```python
from build123d import *

# Parameters (mm, degrees)
SKETCH1_R           = 2.25
BOSS_EXTRUDE1_DEPTH = 3
BOSS_EXTRUDE2_DEPTH = 40
BOSS_EXTRUDE3_START = -2
BOSS_EXTRUDE3_DEPTH = 3
SKETCH6_R           = 1.5
CUT_EXTRUDE1_DEPTH  = 39
FILLET1_R           = 2


with BuildPart() as part:
    # Sketch1 → Boss-Extrude1 (new body)
    with BuildSketch(Plane(origin=(0, 0, 0), x_dir=(1, 0, 0), z_dir=(0, 1, 0))):
        with BuildLine():
            Line((41.207095158, 87.944444444), (68.081287652, 33.777777778))
            ThreePointArc((68.081287652, 33.777777778), (0, -76), (-68.081287652, 33.777777778))
            Line((-68.081287652, 33.777777778), (-41.207095158, 87.944444444))
            ThreePointArc((-41.207095158, 87.944444444), (0, 113.5), (41.207095158, 87.944444444))
        make_face()
        with Locations((40, 67.5)):
            Circle(SKETCH1_R, mode=Mode.SUBTRACT)
        with Locations((70, 0)):
            Circle(SKETCH1_R, mode=Mode.SUBTRACT)
        with Locations((56.631189606, -41.14496766)):
            Circle(SKETCH1_R, mode=Mode.SUBTRACT)
        with Locations((21.631189606, -66.573956141)):
            Circle(SKETCH1_R, mode=Mode.SUBTRACT)
        with Locations((-21.631189606, -66.573956141)):
            Circle(SKETCH1_R, mode=Mode.SUBTRACT)
        with Locations((-56.631189606, -41.14496766)):
            Circle(SKETCH1_R, mode=Mode.SUBTRACT)
        with Locations((-70, 0)):
            Circle(SKETCH1_R, mode=Mode.SUBTRACT)
        with Locations((28.284271247, 95.784271247)):
            Circle(SKETCH1_R, mode=Mode.SUBTRACT)
        with Locations((0, 107.5)):
            Circle(SKETCH1_R, mode=Mode.SUBTRACT)
        with Locations((-28.284271247, 95.784271247)):
            Circle(SKETCH1_R, mode=Mode.SUBTRACT)
        with Locations((-40, 67.5)):
            Circle(SKETCH1_R, mode=Mode.SUBTRACT)
        with Locations((-50.153461651, 44.654711284)):
            Circle(SKETCH1_R, mode=Mode.SUBTRACT)
        with Locations((-60.306923303, 21.809422569)):
            Circle(SKETCH1_R, mode=Mode.SUBTRACT)
        with Locations((50.153461651, 44.654711284)):
            Circle(SKETCH1_R, mode=Mode.SUBTRACT)
        with Locations((60.306923303, 21.809422569)):
            Circle(SKETCH1_R, mode=Mode.SUBTRACT)
        with BuildLine():
            ThreePointArc((28.511087055, 79.67037037), (0, 98.5), (-28.511087055, 79.67037037))
            Line((-28.511087055, 79.67037037), (-52.883467924, 22.574074074))
            ThreePointArc((-52.883467924, 22.574074074), (0, -57.5), (52.883467924, 22.574074074))
            Line((52.883467924, 22.574074074), (28.511087055, 79.67037037))
        make_face(mode=Mode.SUBTRACT)
    extrude(amount=BOSS_EXTRUDE1_DEPTH)

    # Sketch1_3 → Boss-Extrude2 (add)
    with BuildSketch(Plane(origin=(0, 0, 0), x_dir=(1, 0, 0), z_dir=(0, 1, 0))):
        with BuildLine():
            Line((28.511087055, 79.67037037), (52.883467924, 22.574074074))
            ThreePointArc((52.883467924, 22.574074074), (0, -57.5), (-52.883467924, 22.574074074))
            Line((-52.883467924, 22.574074074), (-28.511087055, 79.67037037))
            ThreePointArc((-28.511087055, 79.67037037), (0, 98.5), (28.511087055, 79.67037037))
        make_face()
        with BuildLine():
            ThreePointArc((25.751949598, 78.492592593), (0, 95.5), (-25.751949598, 78.492592593))
            Line((-25.751949598, 78.492592593), (-50.124330467, 21.396296296))
            ThreePointArc((-50.124330467, 21.396296296), (0, -54.5), (50.124330467, 21.396296296))
            Line((50.124330467, 21.396296296), (25.751949598, 78.492592593))
        make_face(mode=Mode.SUBTRACT)
    extrude(amount=BOSS_EXTRUDE2_DEPTH)

    # Sketch5 → Boss-Extrude3 (add)
    with BuildSketch(Plane(origin=(0, 40, 0), x_dir=(1, 0, 0), z_dir=(0, 1, 0)).offset(BOSS_EXTRUDE3_START)):
        with BuildLine():
            Line((25.751949598, 78.492592593), (50.124330467, 21.396296296))
            ThreePointArc((50.124330467, 21.396296296), (0, -54.5), (-50.124330467, 21.396296296))
            Line((-50.124330467, 21.396296296), (-25.751949598, 78.492592593))
            ThreePointArc((-25.751949598, 78.492592593), (0, 95.5), (25.751949598, 78.492592593))
        make_face()
        with BuildLine():
            Line((-20.233674684, 76.137037037), (-44.606055554, 19.040740741))
            ThreePointArc((-44.606055554, 19.040740741), (0, -48.5), (44.606055554, 19.040740741))
            Line((44.606055554, 19.040740741), (20.233674684, 76.137037037))
            ThreePointArc((20.233674684, 76.137037037), (0, 89.5), (-20.233674684, 76.137037037))
        make_face(mode=Mode.SUBTRACT)
    extrude(amount=-BOSS_EXTRUDE3_DEPTH)

    # Sketch6 → Cut-Extrude1 (cut, through all)
    with BuildSketch(Plane(origin=(0, 38, 0), x_dir=(1, 0, 0), z_dir=(0, 1, 0))):
        with Locations((0, -51)):
            Circle(SKETCH6_R)
        with Locations((0, 92)):
            Circle(SKETCH6_R)
        with Locations((14.052622691, 87.569225085)):
            Circle(SKETCH6_R)
        with Locations((23.022469209, 75.879493511)):
            Circle(SKETCH6_R)
        with Locations((21.553531349, -46.221697139)):
            Circle(SKETCH6_R)
        with Locations((39.068266599, -32.782168094)):
            Circle(SKETCH6_R)
        with Locations((49.262217141, -13.1997713)):
            Circle(SKETCH6_R)
        with Locations((50.225195404, 8.856057061)):
            Circle(SKETCH6_R)
        with Locations((27.835315177, 65.055939465)):
            Circle(SKETCH6_R)
        with Locations((33.935175216, 51.257307943)):
            Circle(SKETCH6_R)
        with Locations((40.035035255, 37.45867642)):
            Circle(SKETCH6_R)
        with Locations((46.134895294, 23.660044897)):
            Circle(SKETCH6_R)
        with Locations((-46.134895294, 23.660044897)):
            Circle(SKETCH6_R)
        with Locations((-40.035035255, 37.45867642)):
            Circle(SKETCH6_R)
        with Locations((-33.935175216, 51.257307943)):
            Circle(SKETCH6_R)
        with Locations((-27.835315177, 65.055939465)):
            Circle(SKETCH6_R)
        with Locations((-50.225195404, 8.856057061)):
            Circle(SKETCH6_R)
        with Locations((-49.262217141, -13.1997713)):
            Circle(SKETCH6_R)
        with Locations((-39.068266599, -32.782168094)):
            Circle(SKETCH6_R)
        with Locations((-21.553531349, -46.221697139)):
            Circle(SKETCH6_R)
        with Locations((-23.022469209, 75.879493511)):
            Circle(SKETCH6_R)
        with Locations((-14.052622691, 87.569225085)):
            Circle(SKETCH6_R)
    extrude(amount=-CUT_EXTRUDE1_DEPTH, mode=Mode.SUBTRACT)

    # Fillet1
    fillet1_edges = [part.edges().sort_by_distance(p)[0] for p in [
        (40.69727749, 3, -51.122222222),
        (0, 3, 57.5),
        (-40.69727749, 3, -51.122222222),
        (0, 3, -98.5),
    ]]
    fillet(fillet1_edges, radius=FILLET1_R)


solid = part.part
```
Model file for the job. Use its own axes, mm. A direction names the side the tool comes from. Coordinates: 2 decimals unless noted, no trailing zeros. Write each loop counter-clockwise with the first axis right and the second up, starting at its lowest first coordinate (ties: lowest second). Pieces come first, ordered by that corner, then holes. Notation, with made-up numbers: (53, 47.25) - (60, 47.25) arc R28 cw to (60, 85.25) - close; hole circle Ø10 at (8.5, -19). An arc over 180 degrees is marked (long way). Use a Markdown table: item, result. Add a question column.
Item 1: 3-axis set-ups, long thin cutter, end or side, ignore diameter. For faces 4 (the face through (38.11, 38.99, -49.54)), 5 (the face through (32.59, 36.52, -47.19)), 6 (the face through (38.11, 17.26, -49.54)), 7 (the face through (40.527, 22.255, -51.522)): which of +Z, -Z, +X, -X, +Y, -Y reach the whole face in a straight line?
Item 2: Band-saw the part on A-A, the plane y = 20. Write the cut outline in (x, z), and give its area (3 significant figures).
Item 3: Drop flat-ended pins along their axis: pin 1 (6 mm diameter, centred on y = 14.5, z = 22.5, fed in from -X); pin 2 (3 mm diameter, centred on y = 23.5, z = -55.5, fed in from -X); pin 3 (6 mm diameter, centred on y = 27.5, z = 4, fed in from +X); pin 4 (2.5 mm diameter, centred on x = -60.31, z = -21.81, fed in from +Y). Give the stop position or say it passes through.
Item 4: Two-plate mould, pull along Z, no slides. Class faces 1 (the face through (1.59, 22.26, 57.48)), 2 (the face through (48.368, 1.479, -43.286)), 3 (the face through (-41.39, 3.6, -50.95)): pulls with the +Z half, pulls with the -Z half, needs draft (parallel to the pull), parting line crosses it, or undercut.
Item 5: Drill centre lines: line 1 along X through (y, z) = (18.5, -5.5); line 2 along Z through (x, y) = (-29.5, 22.5); line 3 along X through (y, z) = (16, -39). Where is each one in solid material? Low to high.
A:
| question | item | result |
|---|---|---|
| 1 | face 4 | +Y |
| 1 | face 5 | +Y, -Y |
| 1 | face 6 | -Y |
| 1 | face 7 | -Z, +X, +Y |
| 2 | outline | (-52.88, -22.57) - (-28.51, -79.67) arc R31 ccw to (28.51, -79.67) - (52.88, -22.57) arc R57.5 ccw (long way) to start; hole (-50.12, -21.4) - (-25.75, -78.49) arc R28 ccw to (25.75, -78.49) - (50.12, -21.4) arc R54.5 ccw (long way) to start |
| 2 | area | 1,240 mm² |
| 3 | pin 1 | stops at x = -54.09 |
| 3 | pin 2 | stops at x = -39.47 |
| 3 | pin 3 | stops at x = 57.49 |
| 3 | pin 4 | passes through |
| 4 | face 1 | parting line crosses it |
| 4 | face 2 | undercut |
| 4 | face 3 | pulls with the -Z half |
| 5 | line 1 | x = -57.24 to -54.22, 54.22 to 57.24 |
| 5 | line 2 | z = -77.35 to -69.71, 45.83 to 49.36 |
| 5 | line 3 | x = -45.87 to -42.61, 42.61 to 45.87 |
